from build123d import *

# Parameters (mm, degrees)
CROQUIS1_R              = 14.1
CROQUIS1_R_2            = 11.1
SALIENTE_EXTRUIR1_DEPTH = 2
CORTAR_EXTRUIR1_DEPTH   = 1


with BuildPart() as part:
    # Croquis1 → Saliente-Extruir1 (new body)
    with BuildSketch(Plane.XY):
        Circle(CROQUIS1_R)
        Circle(CROQUIS1_R_2, mode=Mode.SUBTRACT)
    extrude(amount=SALIENTE_EXTRUIR1_DEPTH)

    # Croquis4 → Revolución1 (revolve)
    with BuildSketch(Plane(origin=(0, 0, 0), x_dir=(1, 0, 0), z_dir=(0, 1, 0))):
        with BuildLine():
            Line((14.1, -2), (14.1, 0))
            Line((14.1, 0), (14.1, 8.1))
            ThreePointArc((14.1, 8.1), (13.8, 8.4), (14.1, 8.7))
            Line((14.1, 8.7), (14.1, 10.1))
            Line((14.1, 10.1), (19.6, 10.1))
            Line((19.6, 10.1), (19.6, 6.55))
            ThreePointArc((19.6, 6.55), (17.1, 4.05), (19.6, 1.55))
            Line((19.6, 1.55), (19.6, -2))
            Line((19.6, -2), (14.1, -2))
        make_face()
    revolve(axis=Axis((0, 0, 0), (0, 0, -1)))

    # Croquis7 → Cortar-Extruir1 (cut)
    with BuildSketch(Plane(origin=(0, 0, -10.1), x_dir=(-1, 0, 0), z_dir=(0, 0, -1))):
        Polygon((14.592528054, 6.692949192), (16.092528054, 9.291025404), (13.092528054, 9.291025404), align=None)
        Polygon((1.5, 15.983974596), (0, 18.582050808), (-1.5, 15.983974596), align=None)
        Polygon((13.092528054, -9.291025404), (16.092528054, -9.291025404), (14.592528054, -6.692949192), align=None)
        Polygon((-1.5, -15.983974596), (0, -18.582050808), (1.5, -15.983974596), align=None)
        Polygon((-14.592528054, -6.692949192), (-16.092528054, -9.291025404), (-13.092528054, -9.291025404), align=None)
        Polygon((-13.092528054, 9.291025404), (-16.092528054, 9.291025404), (-14.592528054, 6.692949192), align=None)
    extrude(amount=-CORTAR_EXTRUIR1_DEPTH, mode=Mode.SUBTRACT)


solid = part.part
CAD build for the part. Positions are in the model's coordinates, mm. A direction names the side the tool comes from. Coordinates: 2 decimals unless noted, no trailing zeros. Loops run counter-clockwise (first coordinate to the right, second up) from the corner with the lowest first, then second, coordinate; pieces in that order, holes last. Notation, with made-up numbers: (54, 48.25) - (81, 48.25) arc R13 cw to (81, 54.25) - close; hole circle Ø8 at (3, -23). An arc over 180 degrees is marked (long way). Write item = value, one per line. Start each with the question number.
Q1. Which spindle directions (+Z, -Z, +X, -X, +Y, -Y) get a long thin tool onto all of the face, cutting with end or side? Do faces 1 (the cylindrical face through (6.506, 12.509, -4.107)), 2 (the cylindrical face through (5.97, 9.36, 0.99)), 3 (the flat face through (13.853, 7.974, -9.607)). Say none if no direction does.
Q2. Drill centre lines: L1, parallel to X at y = 0.5, z = -9; L2, parallel to Y at x = 0, z = -1.25; L3, parallel to Y at x = 0, z = 1.1. Where is each one in solid material? Low to high.
Q3. Cut at B-B, the plane z = -5.75. List the corners of the cut face in (x, y).
Q4. Flat gauge pins, fed straight in: pin 1 Ø4 at (x, z) = (14.5, -4) entering from -Y; pin 2 Ø0.8 at (x, z) = (-0.5, -9.5) entering from +Y; pin 3 Ø0.8 at (x, y) = (0.5, 17) entering from -Z; pin 4 Ø2 at (y, z) = (-8.5, 0.5) entering from -X. Where does each tip first touch, or does it go through?
Q5. Pull direction Y, two halves, no side cores. Call faces 4 (the cylindrical face through (-4.249, 19.134, 0.25)), 5 (the flat face through (-0.76, 17.265, -9.607)), 6 (the flat face through (0.1, 14.4, -10.1)): pulls with the +Y half, pulls with the -Y half, needs draft (parallel to the pull), parting line crosses it, or undercut.
Q6. Cut at A-A, the plane y = 0. List the corners of the cut face in (x, z).
Computed:
q1.face_1 = none
q1.face_2 = +Z, -Z
q1.face_3 = -Z
q2.L1 = -19.59 to -14.09, 14.09 to 19.59
q2.L2 = -19.6 to -14.1, 14.1 to 19.6
q2.L3 = -19.6 to -11.1, 11.1 to 19.6
q3.outline = circle Ø35.53 at (0, 0); hole circle Ø28.2 at (0, 0)
q4.pin_1 = -11.73
q4.pin_2 = 19.6
q4.pin_3 = -10.1
q4.pin_4 = -18.11
q5.face_4 = parting line crosses it
q5.face_5 = undercut
q5.face_6 = needs draft
q6.outline = (-19.6, -10.1) - (-14.1, -10.1) - (-14.1, -8.7) arc R0.3 ccw to (-14.1, -8.1) - (-14.1, 0) - (-11.1, 0) - (-11.1, 2) - (-19.6, 2) - (-19.6, -1.55) arc R2.5 cw to (-19.6, -6.55) - close; (11.1, 0) - (14.1, 0) - (14.1, -8.1) arc R0.3 ccw to (14.1, -8.7) - (14.1, -10.1) - (19.6, -10.1) - (19.6, -6.55) arc R2.5 cw to (19.6, -1.55) - (19.6, 2) - (11.1, 2) - close
